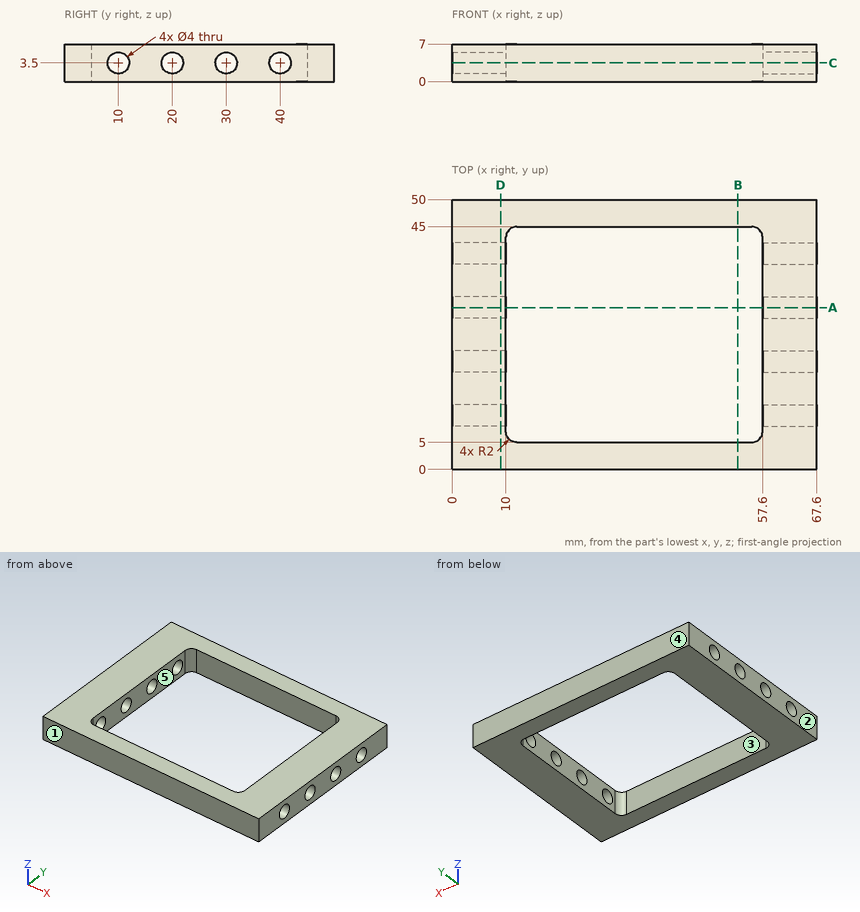
Verification items for this drawing (mm, ordinates from the low corner). A direction names the side the tool comes from. Coordinates: 2 decimals unless noted, no trailing zeros. Order: outer loops, then holes, each group sorted by start corner. A loop starts at its lowest first (then second) coordinate and runs counter-clockwise, first axis right, second up.
Q1. Draft check along Y on the marked faces 1, 2 and 3. Enter one of: released by +Y, released by -Y, zero draft, split by the parting line, or undercut.
Reply:
face 1: released by -Y
face 2: zero draft
face 3: undercut
Q2. Thickness scan on probe 1 along Y at (x, z) = (63.25, 3.5); probe 2 along Y at (x, z) = (29, 2.5); probe 3 along X at (y, z) = (34.5, 5.75). Record the ranges inside material, lowest first.
Reply:
probe 1: y = 0 to 8, 12 to 18, 22 to 28, 32 to 38, 42 to 50
probe 2: y = 0 to 5, 45 to 50
probe 3: x = 0 to 10, 57.6 to 67.6
Q3. Sectioned sample at B-B on x = 53. Record the cut outline in (y, z).
Reply:
outline: (0, 0) - (5, 0) - (5, 7) - (0, 7) - close; (45, 0) - (50, 0) - (50, 7) - (45, 7) - close
Q4. Sectioned sample at C-C on z = 3.5. Give the number of separate pieces and of enclosed holes in the cut face, and give its area (3 significant figures).
Reply:
separate pieces: 8
enclosed holes: 0
area: 1,160 mm2
Q5. Sectioned sample at D-D on x = 9. Record the cut outline in (y, z).
Reply:
outline: (0, 0) - (50, 0) - (50, 7) - (0, 7) - close; hole circle Ø4 at (10, 3.5); hole circle Ø4 at (20, 3.5); hole circle Ø4 at (30, 3.5); hole circle Ø4 at (40, 3.5)
Q6. Tool access check on the marked faces 4 and 5. Record the directions out of +Z, -Z, +X, -X, +Y, -Y that give a thin tool (end or side, any length) a straight path to the whole face; none if there is none.
Reply:
face 4: +Z, -Z, +X, -X, +Y
face 5: +Z, -Z
Q7. Sectioned sample at A-A on y = 30. Record the cut outline in (x, z), and give its area (3 significant figures).
Reply:
outline: (0, 0) - (10, 0) - (10, 1.5) - (0, 1.5) - close; (0, 5.5) - (10, 5.5) - (10, 7) - (0, 7) - close; (57.6, 0) - (67.6, 0) - (67.6, 1.5) - (57.6, 1.5) - close; (57.6, 5.5) - (67.6, 5.5) - (67.6, 7) - (57.6, 7) - close
area: 60.0 mm2
Q8. Depth check by flat-ended pin: pin 1 Ø2 at (x, z) = (45.5, 3) entering from -Y. Enter the tip coordinate at first touch or a pass-through.
Reply:
pin 1: stops at y = 0
